The listing builds one solid part. Answer for the finished solid, in the listing's coordinates (mm). A direction names the side the tool comes from. Round coordinates to 2 decimals unless told otherwise and drop trailing zeros. Loops run counter-clockwise (first coordinate to the right, second up) from the corner with the lowest first, then second, coordinate; pieces in that order, holes last. Notation, with made-up numbers: (60, -15) -> (72, -15) arc R13 ccw to (72, 6) -> close; hole circle Ø6 at (83.5, 23). An arc over 180 degrees is marked (long way). Write each question's results on one line, items separated by ' | '. Start each with the question number.
(1) For faces 1 (the face through (29.15, -3, 6)), 2 (the face through (22.49, 23.26, 50.87)), 3 (the face through (21, -3, 12)), determine the directions among +Z, -Z, +X, -X, +Y, -Y from which every point of the face is accessible in a straight line to the end or side of a thin tool.
(2) Flat-ended cylindrical pins translate along their axes: pin 1 (5 mm diameter, centred on y = 1, z = 44.5, fed in from -X); pin 2 (2 mm diameter, centred on y = -4, z = 4.5, fed in from -X); pin 3 (5 mm diameter, centred on x = 18, y = -2, fed in from +Z). Find the tip coordinate at first contact, or state that the pin passes through.
(3) The part is cut by section D-D (y = 27). Determine the outline of the cut face in (x, z).
(4) The part is cut by section C-C (x = 21.15). Determine the outline of the cut face in (y, z), plus the area to 3 significant figures.
(5) The part is cut by section A-A (y = 21.15). Determine the outline of the cut face in (x, z), plus the area to 3 significant figures.
(6) Straight lines are drawn through the part: probe 1 along X at (y, z) = (5.65, 38.5); probe 2 along Y at (x, z) = (5, 38). For each, find the intervals that lie inside material, in ascending order.
(7) The part is cut by section B-B (z = 18). Determine the outline of the cut face in (x, y).
(8) Determine the mould class of faces 4 (the face through (6.83, 6.73, 37.72)), 5 (the face through (37.83, 6.73, 37.72)), 6 (the face through (0, 21, 20)), 7 (the face through (21, -6.5, 6)) for opening direction Y: released by +Y, released by -Y, zero draft, split by the parting line, or undercut.
```python
from build123d import *

# Parameters (mm, degrees)
F0_W      = 42.3
F0_H      = 42.3
F1_DEPTH  = 40
F3_D      = 3.2
F3_DEPTH  = 4.5
F3_TIP    = 0.9613769904
F4_R      = 11
F5_DEPTH  = 2
F6_R      = 2.5
F7_DEPTH  = 18
F8_SIZE   = 5
F9_W      = 16
F9_H      = 12
F10_DEPTH = 6.5


with BuildPart() as f1:
    # F0 (on Top) → F1 (new body)
    with BuildSketch(Plane.XY):
        with Locations((21.15, 21.15)):
            Rectangle(F0_W, F0_H)
    extrude(amount=F1_DEPTH)

    # F3
    with Locations(Plane.XY.offset(40)):
        with Locations((5.65, 36.65), (36.65, 36.65), (5.65, 5.65), (36.65, 5.65)):
            Hole(F3_D / 2, depth=F3_DEPTH)
            with Locations((0, 0, -(F3_DEPTH + F3_TIP / 2))):  # 118° drill point
                Cone(0, F3_D / 2, F3_TIP, mode=Mode.SUBTRACT)

    # F4 (on face) → F5 (join)
    with BuildSketch(Plane.XY.offset(40)):
        with Locations((21.15, 21.15)):
            Circle(F4_R)
    extrude(amount=F5_DEPTH)

    # F6 (on face) → F7 (join)
    with BuildSketch(Plane.XY.offset(42)):
        with Locations((21.15, 21.15)):
            Circle(F6_R)
    extrude(amount=F7_DEPTH)

    # F8
    f8_edges = [f1.edges().sort_by_distance(p)[0] for p in [
        (42.3, 42.3, 20),
        (42.3, 0, 20),
        (0, 42.3, 20),
        (0, 0, 20),
    ]]
    chamfer(f8_edges, length=F8_SIZE)

    # F9 (on face) → F10 (join)
    with BuildSketch(Plane.XZ):
        with Locations((21.15, 6)):
            Rectangle(F9_W, F9_H)
    extrude(amount=F10_DEPTH)


solid = f1.part
```
Checked values:
1) face 1: +Z, -Z, +X, -Y | face 2: +Z | face 3: +Z, +X, -X, -Y
2) pin 1: passes through | pin 2: stops at x = 13.15 | pin 3: stops at z = 40
3) outline: (0, 0) -> (42.3, 0) -> (42.3, 40) -> (30.47, 40) -> (30.47, 42) -> (11.83, 42) -> (11.83, 40) -> (0, 40) -> close
4) outline: (-6.5, 0) -> (42.3, 0) -> (42.3, 40) -> (32.15, 40) -> (32.15, 42) -> (23.65, 42) -> (23.65, 60) -> (18.65, 60) -> (18.65, 42) -> (10.15, 42) -> (10.15, 40) -> (0, 40) -> (0, 12) -> (-6.5, 12) -> close | area: 1,900 mm2
5) outline: (0, 0) -> (42.3, 0) -> (42.3, 40) -> (32.15, 40) -> (32.15, 42) -> (23.65, 42) -> (23.65, 60) -> (18.65, 60) -> (18.65, 42) -> (10.15, 42) -> (10.15, 40) -> (0, 40) -> close | area: 1,830 mm2
6) probe 1: x = 0 to 4.05, 7.25 to 35.05, 38.25 to 42.3 | probe 2: y = 0 to 4.19, 7.11 to 35.19, 38.11 to 42.3
7) outline: (0, 5) -> (5, 0) -> (37.3, 0) -> (42.3, 5) -> (42.3, 37.3) -> (37.3, 42.3) -> (5, 42.3) -> (0, 37.3) -> close
8) face 4: undercut | face 5: undercut | face 6: zero draft | face 7: released by -Y
